from build123d import *

# Parameters (mm, degrees)
SKETCH1_W           = 21
SKETCH1_H           = 24
BOSS_EXTRUDE1_DEPTH = 2
SKETCH2_W           = 18.6
SKETCH2_H           = 22
BOSS_EXTRUDE2_DEPTH = 13.2
SKETCH3_W           = 4.885548906
SKETCH3_H           = 0.896605201
SKETCH3_H_2         = 0.661547926
SKETCH3_W_2         = 6.515688333
BOSS_EXTRUDE3_DEPTH = 6.3
BOSS_EXTRUDE4_DEPTH = 10


with BuildPart() as part:
    # Sketch1 → Boss-Extrude1 (new body)
    with BuildSketch(Plane(origin=(0, 0, 0), x_dir=(1, 0, 0), z_dir=(0, 1, 0))):
        Rectangle(SKETCH1_W, SKETCH1_H)
    extrude(amount=BOSS_EXTRUDE1_DEPTH)

    # Sketch2 → Boss-Extrude2 (add)
    with BuildSketch(Plane.XZ):
        Rectangle(SKETCH2_W, SKETCH2_H)
    extrude(amount=BOSS_EXTRUDE2_DEPTH)

    # Sketch3 → Boss-Extrude3 (add)
    with BuildSketch(Plane.XZ.offset(13.2)):
        with Locations((4.472159413, 2.304982967)):
            Rectangle(SKETCH3_W, SKETCH3_H)
        with Locations((4.472159413, -6.706929347)):
            Rectangle(SKETCH3_W, SKETCH3_H_2)
        with Locations((-4.244383184, -6.706929347)):
            Rectangle(SKETCH3_W_2, SKETCH3_H_2)
        with Locations((-4.244383184, 2.304982967)):
            Rectangle(SKETCH3_W_2, SKETCH3_H)
    extrude(amount=BOSS_EXTRUDE3_DEPTH)

    # Sketch4 → Boss-Extrude4 (add, symmetric)
    with BuildSketch(Plane.XY):
        Polygon((-8.803379904, 1.907067214), (7.189360766, 7.787523085), (9.380607332, 1.828114693), align=None)
    extrude(amount=BOSS_EXTRUDE4_DEPTH, both=True)


solid = part.part
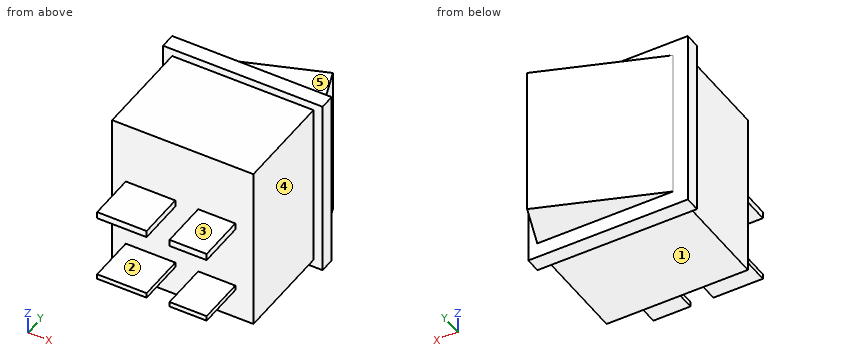
Could you check a few things on this model? Use its own coordinates, in mm. Face numbers are marked on the shaded views. A direction names the side the tool comes from. Coordinates: 2 decimals unless noted, no trailing zeros. Loops run counter-clockwise (first coordinate to the right, second up) from the corner with the lowest first, then second, coordinate; pieces in that order, holes last.
1. For P1, Ø3, axis at x = -3.5, y = -15, coming from the -Z side; P2, Ø5, axis at x = -4, y = -18, coming from the +Z side; P3, Ø4, axis at x = 4, y = -3.5, coming from the +Z side; P4, Ø1, axis at x = -4.5, y = 4.5, coming from the -Z side, each with a flat end and sliding along its axis, tell me the tip position at first contact or that it passes through.
2. For the marked faces 1, 2, 3, 4 and 5, which set-ups out of +Z, -Z, +X, -X, +Y, -Y let a thin tool reach every point of the face, with its end or its side?
3. Imagine slicing it at C-C (x = -2.25). Please give me the cut outline in (y, z), and give its area (3 significant figures).
4. Imagine slicing it at B-B (z = -3). Please give me the cut outline in (x, y).
5. Imagine slicing it at A-A (y = -17.5). Please give me the cut outline in (x, z).
6. I need wall thicknesses on L1, parallel to Z at x = 3.75, y = -14; L2, parallel to Y at x = 5.5, z = -10.5; L3, parallel to Z at x = -3.5, y = -2. Which ranges of each line are inside material? Lowest first, please.
7. Imagine slicing it at D-D (y = -5.5). Please give me the cut outline in (x, z), and give its area (3 significant figures).
Computed values:
1. P1: stops at z = -7.04
1. P2: stops at z = 2.75
1. P3: stops at z = 11
1. P4: passes through
2. face 1: -Z, +X, -X, -Y
2. face 2: +X, -X, -Y
2. face 3: +Z, +X, -X, -Y
2. face 4: +Z, -Z, +X, -Y
2. face 5: +Z, +X, -X, +Y
3. outline: (-19.5, -7.04) - (-13.2, -7.04) - (-13.2, -11) - (0, -11) - (0, -12) - (2, -12) - (2, -10) - (4.32, -10) - (4.32, 10) - (2, 10) - (2, 12) - (0, 12) - (0, 11) - (-13.2, 11) - (-13.2, 2.75) - (-19.5, 2.75) - (-19.5, 1.86) - (-13.2, 1.86) - (-13.2, -6.38) - (-19.5, -6.38) - close
3. area: 395 mm2
4. outline: (-10.5, 0) - (-9.3, 0) - (-9.3, -13.2) - (9.3, -13.2) - (9.3, 0) - (10.5, 0) - (10.5, 2) - (9.32, 2) - (7.19, 7.79) - (-8.55, 2) - (-10.5, 2) - close
5. outline: (-7.5, -7.04) - (-0.99, -7.04) - (-0.99, -6.38) - (-7.5, -6.38) - close; (-7.5, 1.86) - (-0.99, 1.86) - (-0.99, 2.75) - (-7.5, 2.75) - close; (2.03, -7.04) - (6.91, -7.04) - (6.91, -6.38) - (2.03, -6.38) - close; (2.03, 1.86) - (6.91, 1.86) - (6.91, 2.75) - (2.03, 2.75) - close
6. L1: z = -7.04 to -6.38, 1.86 to 2.75
6. L2: y = -13.2 to 2
6. L3: z = -11 to 11
7. outline: (-9.3, -11) - (9.3, -11) - (9.3, 11) - (-9.3, 11) - close
7. area: 409 mm2
